Could you check a few things on this model? Use its own coordinates, in mm. A direction names the side the tool comes from. Coordinates: 2 decimals unless noted, no trailing zeros. Loops run counter-clockwise (first coordinate to the right, second up) from the corner with the lowest first, then second, coordinate; pieces in that order, holes last.
from build123d import *

# Parameters (mm, degrees)
SKETCH2_W           = 60
SKETCH2_H           = 60
BOSS_EXTRUDE1_DEPTH = 42
SKETCH3_W           = 60
SKETCH3_H           = 60
BOSS_EXTRUDE2_DEPTH = 38
FILLET1_R           = 5
FILLET2_R           = 5
FILLET3_R           = 5
SKETCH4_R           = 2.25
CUT_EXTRUDE1_DEPTH  = 10
SKETCH5_R           = 12
BOSS_EXTRUDE3_DEPTH = 4
SKETCH6_R           = 5
BOSS_EXTRUDE4_DEPTH = 28
CUT_EXTRUDE2_DEPTH  = 28
SKETCH8_W           = 83.4072332
SKETCH8_H           = 75.183984856
CUT_EXTRUDE3_DEPTH  = 84
SKETCH9_R           = 5
BOSS_EXTRUDE5_DEPTH = 5


with BuildPart() as part:
    # Sketch2 → Boss-Extrude1 (new body)
    with BuildSketch(Plane.XY):
        with Locations((30, 30)):
            Rectangle(SKETCH2_W, SKETCH2_H)
    extrude(amount=BOSS_EXTRUDE1_DEPTH)

    # Fillet1
    fillet1_edges = [part.edges().sort_by_distance(p)[0] for p in [
        (0, 60, 21),
        (60, 60, 21),
        (60, 0, 21),
        (0, 0, 21),
    ]]
    fillet(fillet1_edges, radius=FILLET1_R)

    # Fillet3
    fillet3_edges = [part.edges().sort_by_distance(p)[0] for p in [
        (30, 0, 42),
        (0, 30, 42),
        (60, 30, 42),
        (30, 60, 42),
        (58.535533906, 58.535533906, 42),
        (1.464466094, 58.535533906, 42),
        (58.535533906, 1.464466094, 42),
        (1.464466094, 1.464466094, 42),
    ]]
    fillet(fillet3_edges, radius=FILLET3_R)


with BuildPart() as body_2:
    # Sketch3 → Boss-Extrude2 (new body)
    with BuildSketch(Plane(origin=(0, 0, 0), x_dir=(-1, 0, 0), z_dir=(0, 0, -1))):
        with Locations((-30, 30)):
            Rectangle(SKETCH3_W, SKETCH3_H)
    extrude(amount=BOSS_EXTRUDE2_DEPTH)

    # Fillet2
    fillet2_edges = [body_2.edges().sort_by_distance(p)[0] for p in [
        (60, 0, -19),
        (60, 60, -19),
        (0, 60, -19),
        (0, 0, -19),
    ]]
    fillet(fillet2_edges, radius=FILLET2_R)

    # Sketch4 → Cut-Extrude1 (cut)
    with BuildSketch(Plane(origin=(0, 0, -38), x_dir=(-1, 0, 0), z_dir=(0, 0, -1))):
        with Locations((-5.251262658, 54.748737342)):
            Circle(SKETCH4_R)
        with Locations((-54.748737342, 54.748737342)):
            Circle(SKETCH4_R)
        with Locations((-54.748737342, 5.251262658)):
            Circle(SKETCH4_R)
        with Locations((-5.251262658, 5.251262658)):
            Circle(SKETCH4_R)
    extrude(amount=-CUT_EXTRUDE1_DEPTH, mode=Mode.SUBTRACT)

    # Sketch5 → Boss-Extrude3 (add)
    with BuildSketch(Plane(origin=(0, 0, -38), x_dir=(-1, 0, 0), z_dir=(0, 0, -1))):
        with Locations((-30, 40)):
            Circle(SKETCH5_R)
    extrude(amount=BOSS_EXTRUDE3_DEPTH)

    # Sketch6 → Boss-Extrude4 (add)
    with BuildSketch(Plane(origin=(0, 0, -42), x_dir=(-1, 0, 0), z_dir=(0, 0, -1))):
        with Locations((-30, 40)):
            Circle(SKETCH6_R)
    extrude(amount=BOSS_EXTRUDE4_DEPTH)

    # Sketch7 → Cut-Extrude2 (cut)
    with BuildSketch(Plane(origin=(0, 42.5, 0), x_dir=(1, 0, 0), z_dir=(0, 1, 0))):
        with BuildLine():
            Line((28, 47), (28, 70))
            Line((28, 70), (32, 70))
            Line((32, 70), (32, 47))
            ThreePointArc((32, 47), (30, 45), (28, 47))
        make_face()
    extrude(amount=CUT_EXTRUDE2_DEPTH, mode=Mode.SUBTRACT)


with BuildPart() as cut_extrude3_tool:
    # Sketch8 → Cut-Extrude3 (new body)
    with BuildSketch(Plane(origin=(0, 0, -42), x_dir=(-1, 0, 0), z_dir=(0, 0, -1))):
        with Locations((-33.52424929, 30.998537299)):
            Rectangle(SKETCH8_W, SKETCH8_H)
    extrude(amount=-CUT_EXTRUDE3_DEPTH)


with BuildPart() as part_1:
    add(part.part)

    # Cut-Extrude3: cut by cut_extrude3_tool
    add(cut_extrude3_tool.part, mode=Mode.SUBTRACT)


with BuildPart() as body_2_1:
    add(body_2.part)

    # Cut-Extrude3: cut by cut_extrude3_tool
    add(cut_extrude3_tool.part, mode=Mode.SUBTRACT)

    # Sketch9 → Boss-Extrude5 (add)
    with BuildSketch(Plane.XY.offset(-42)):
        with Locations((30, 40)):
            Circle(SKETCH9_R)
    extrude(amount=BOSS_EXTRUDE5_DEPTH)


solid = body_2_1.part
(1) Imagine slicing it at D-D, the plane x = 28.5. Write out the boundary of the cut face in (y, z), and give its area (3 significant figures).
Answers:
outline: (35.23, -70) - (42.5, -70) - (42.5, -45.68) - (44.77, -45.68) - (44.77, -37) - (35.23, -37) - close
area: 260 mm2
(2) Imagine slicing it at A-A, the plane x = 30. Write out the boundary of the cut face in (y, z).
Answers:
outline: (35, -70) - (42.5, -70) - (42.5, -45) - (45, -45) - (45, -37) - (35, -37) - close
(3) For pin 1 (5 mm diameter, centred on x = 26.5, z = -44.5, fed in from +Y); pin 2 (0.6 mm diameter, centred on y = 43.5, z = -57.5, fed in from -X); pin 3 (2 mm diameter, centred on x = 30, z = -57.5, fed in from +Y), each with a flat end and sliding along its axis, tell me the tip position at first contact or that it passes through.
Answers:
pin 1: stops at y = 44.9
pin 2: stops at x = 26.16
pin 3: stops at y = 42.5
(4) Imagine slicing it at C-C, the plane z = -53. Write out the boundary of the cut face in (x, y), and give its area (3 significant figures).
Answers:
outline: (28, 42.5) - (28, 44.58) arc R5 ccw (long way) to (32, 44.58) - (32, 42.5) - close
area: 69.1 mm2
(5) I need wall thicknesses on probe 1 along Y at (x, z) = (30, -66); probe 2 along X at (y, z) = (39.75, -38.5); probe 3 along Y at (x, z) = (31.75, -57). Which ranges of each line are inside material? Lowest first, please.
Answers:
probe 1: y = 35 to 42.5
probe 2: x = 25.01 to 34.99
probe 3: y = 35.32 to 42.5
(6) Imagine slicing it at B-B, the plane y = 43.5. Write out the boundary of the cut face in (x, z), and give its area (3 significant figures).
Answers:
outline: (26.43, -70) - (28, -70) - (28, -47) arc R2 cw to (32, -47) - (32, -70) - (33.57, -70) - (33.57, -37) - (26.43, -37) - close
area: 137 mm2
(7) We'd pull the mould along Z, two halves only. Please class faces 3 (the face through (30, 44, -45)), 4 (the face through (30, 42.5, -58)), 5 (the face through (30, 40, -37)): +Z half, -Z half, draft (parallel to the pull), parting line (faces both ways), or undercut.
Answers:
face 3: -Z half
face 4: draft
face 5: +Z half
(8) Which directions (+Z, -Z, +X, -X, +Y, -Y) give clear straight access to the entire face, cutting with the end or side of a thin tool? Please do faces 1 (the face through (28, 44, -58)), 2 (the face through (30, 40, -70)).
Answers:
face 1: -Z, +Y
face 2: -Z, +X, -X, +Y, -Y
